Print and shaded views of the part. All mm, measured from the part's lowest x, y and z. A direction names the side the tool comes from. Round coordinates to 2 decimals unless told otherwise and drop trailing zeros. Loops run counter-clockwise (first coordinate to the right, second up) from the corner with the lowest first, then second, coordinate; pieces in that order, holes last. Notation, with made-up numbers: (76.25, 73.5) - (133.25, 73.5) arc R22 cw to (133.25, 84.5) - close; hole circle Ø4 at (-3.75, 9). An arc over 180 degrees is marked (long way). Answer as a JSON object with one key per item and string values.
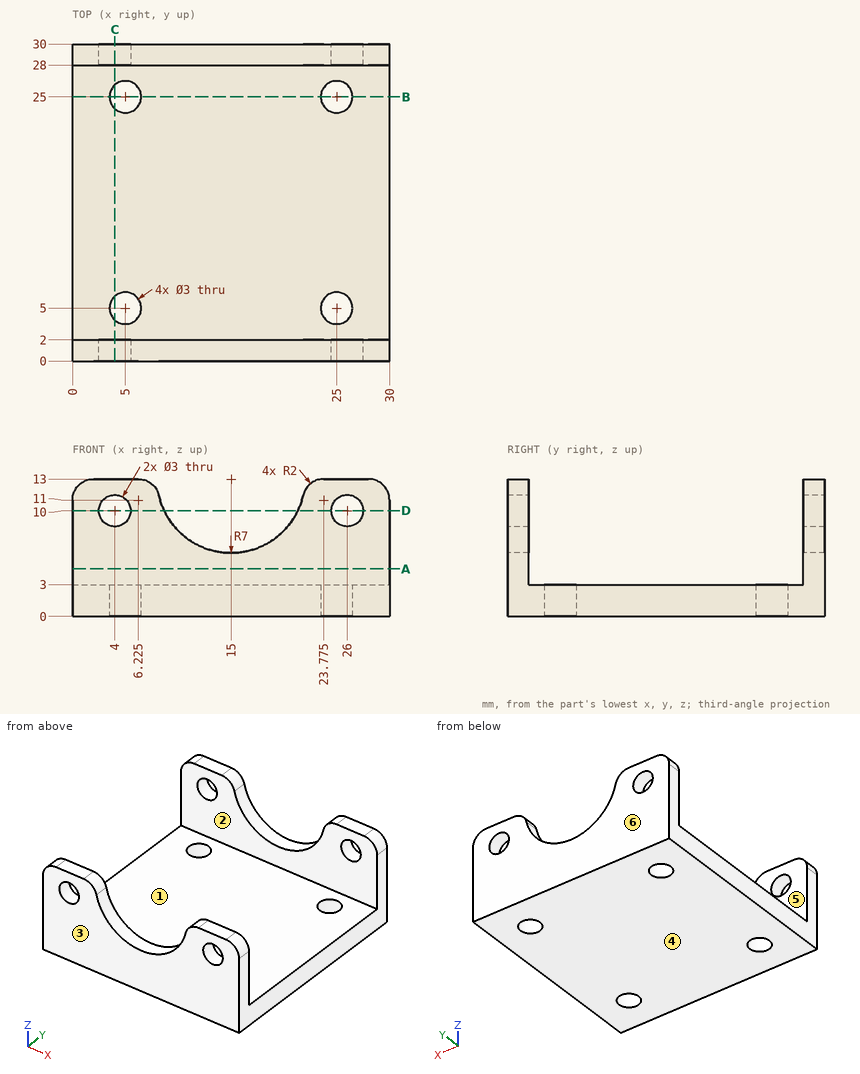
1) Tool access for the marked faces 5 and 6: list every direction of +Z, -Z, +X, -X, +Y, -Y with a clear straight run to the whole face (end or side of a thin tool).
Values follow:
{"face 5": "+Z, +X, -X", "face 6": "+Z, -Z, +X, -X, +Y"}
2) Slice it at B-B on y = 25. List the corners of the cut face in (x, z).
Values follow:
{"outline": "(0, 0) - (3.5, 0) - (3.5, 3) - (0, 3) - close; (6.5, 0) - (23.5, 0) - (23.5, 3) - (6.5, 3) - close; (26.5, 0) - (30, 0) - (30, 3) - (26.5, 3) - close"}
3) Drop a flat-ended pin along its axis: P1, Ø4, axis at x = 25, y = 25, coming from the +Z side. Give the stop position or say it passes through.
Values follow:
{"P1": "z = 3"}
4) Slice it at A-A on z = 4.5. List the corners of the cut face in (x, y), then the cut area to 3 significant figures.
Values follow:
{"outline": "(0, 0) - (30, 0) - (30, 2) - (0, 2) - close; (0, 28) - (30, 28) - (30, 30) - (0, 30) - close", "area": "120 mm²"}
5) Slice it at D-D on z = 10. Count the separate pieces of the cut face and the enclosed holes in it, then the cut area to 3 significant figures.
Values follow:
{"separate pieces": "8", "enclosed holes": "0", "area": "45.4 mm²"}
6) Two-plate mould, pull along Y, no slides. Class the marked faces 1, 2, 3 and 4: pulls with the +Y half, pulls with the -Y half, needs draft (parallel to the pull), parting line crosses it, or undercut.
Values follow:
{"face 1": "undercut", "face 2": "undercut", "face 3": "pulls with the -Y half", "face 4": "needs draft"}
7) Probe probe 1 along Y at (x, z) = (25, 1.9); probe 2 along Y at (x, z) = (6.75, 8.5); probe 3 along Z at (x, y) = (26, 0.8). List the from-to ranges inside material, lowest first.
Values follow:
{"probe 1": "0 to 3.5, 6.5 to 23.5, 26.5 to 30", "probe 2": "0 to 2, 28 to 30", "probe 3": "0 to 8.5, 11.5 to 13"}
8) Slice it at C-C on x = 4. List the corners of the cut face in (y, z), then the cut area to 3 significant figures.
Values follow:
{"outline": "(0, 0) - (3.88, 0) - (3.88, 3) - (2, 3) - (2, 8.5) - (0, 8.5) - close; (0, 11.5) - (2, 11.5) - (2, 13) - (0, 13) - close; (6.12, 0) - (23.88, 0) - (23.88, 3) - (6.12, 3) - close; (26.12, 0) - (30, 0) - (30, 8.5) - (28, 8.5) - (28, 3) - (26.12, 3) - close; (28, 11.5) - (30, 11.5) - (30, 13) - (28, 13) - close", "area": "105 mm²"}
